Part print with two shaded views. Sizes in mm from the minimum x, y, z corner. A direction names the side the tool comes from. Give positions to 0.01 mm unless a question says otherwise; leave off trailing zeros. Loops run counter-clockwise (first coordinate to the right, second up) from the corner with the lowest first, then second, coordinate; pieces in that order, holes last. Notation, with made-up numbers: (57, 23) -> (94, 23) arc R21 cw to (94, 43) -> close; hole circle Ø4 at (25, 87). An arc over 180 degrees is marked (long way). One line per question, with ' | ' between items. Start each with the question number.
(1) Mould opens along X. For the marked faces 1, 2 and 3 say: pulls with the +X half, pulls with the -X half, needs draft (parallel to the pull), parting line crosses it, or undercut.
(2) Drill centre lines: L1, parallel to X at y = 41, z = 44.5; L2, parallel to Y at x = 35.5, z = 53; L3, parallel to Z at x = 20.5, y = 7. Where is each one in solid material? Low to high. Write a range as from..to.
(3) 3-axis set-ups, long thin cutter, end or side, ignore diameter. For the marked faces 4, 5 and 6: which of +Z, -Z, +X, -X, +Y, -Y reach the whole face in a straight line?
(4) Slice it at A-A, the plane y = 12.5. Write the cut outline in (x, z), then the cut area to 3 significant figures.
(5) Slice it at D-D, the plane y = 55. Write the cut outline in (x, z).
(6) Slice it at B-B, the plane x = 34. Write the cut outline in (y, z), then the cut area to 3 significant figures.
(7) Slice it at C-C, the plane z = 26. Write the cut outline in (x, y).
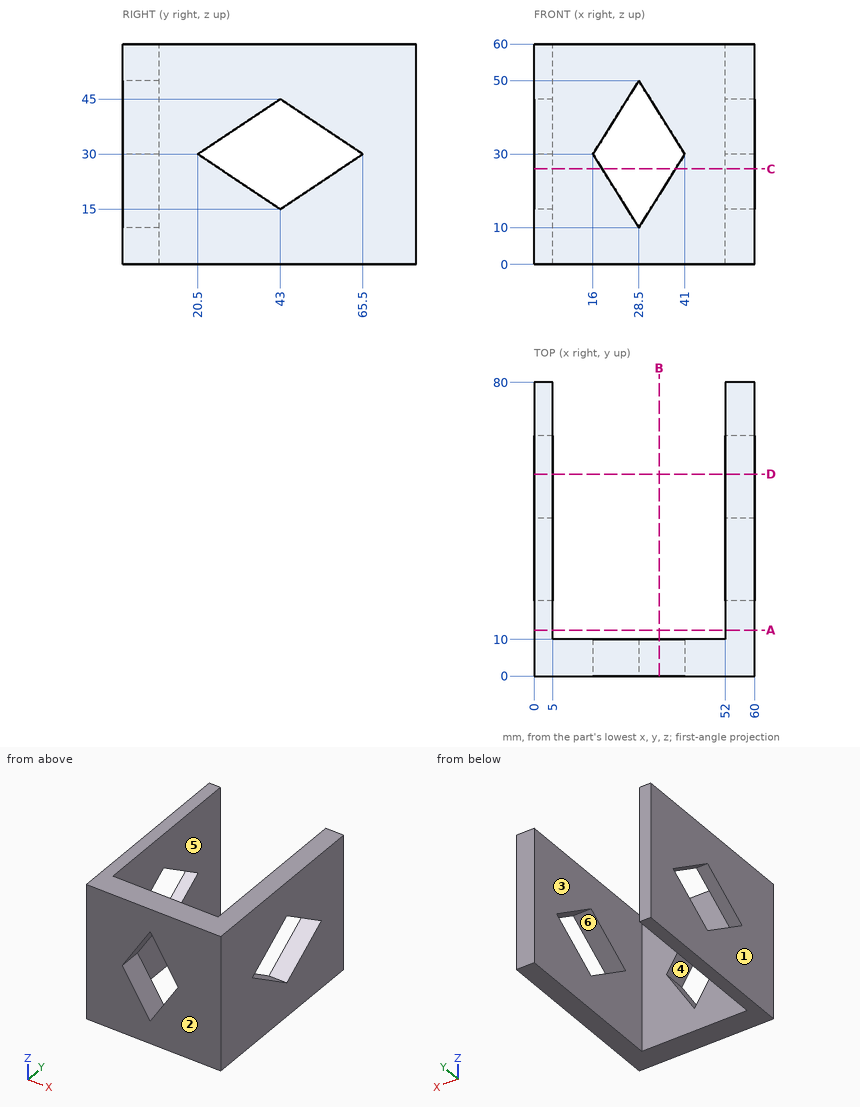
Final values:
1) face 1: pulls with the -X half | face 2: needs draft | face 3: undercut
2) L1: 0..5, 52..60 | L2: 0..10 | L3: 0..22.8, 37.2..60
3) face 4: +Y, -Y | face 5: +Z, -Z, +Y | face 6: +X, -X
4) outline: (0, 0) -> (5, 0) -> (5, 60) -> (0, 60) -> close; (52, 0) -> (60, 0) -> (60, 60) -> (52, 60) -> close | area: 780 mm2
5) outline: (0, 0) -> (5, 0) -> (5, 23) -> (0, 23) -> close; (0, 37) -> (5, 37) -> (5, 60) -> (0, 60) -> close; (52, 0) -> (60, 0) -> (60, 23) -> (52, 23) -> close; (52, 37) -> (60, 37) -> (60, 60) -> (52, 60) -> close
6) outline: (0, 0) -> (10, 0) -> (10, 18.8) -> (0, 18.8) -> close; (0, 41.2) -> (10, 41.2) -> (10, 60) -> (0, 60) -> close | area: 376 mm2
7) outline: (0, 0) -> (18.5, 0) -> (18.5, 10) -> (5, 10) -> (5, 26.5) -> (0, 26.5) -> close; (0, 59.5) -> (5, 59.5) -> (5, 80) -> (0, 80) -> close; (38.5, 0) -> (60, 0) -> (60, 26.5) -> (52, 26.5) -> (52, 10) -> (38.5, 10) -> close; (52, 59.5) -> (60, 59.5) -> (60, 80) -> (52, 80) -> close
